Verification items for the finished model (mm, model axes). Coordinates: 2 decimals unless noted, no trailing zeros. Write each loop counter-clockwise with the first axis right and the second up, starting at its lowest first coordinate (ties: lowest second). Pieces come first, ordered by that corner, then holes. Notation, with made-up numbers: M -39,40 L -13,40 A6 ccw -13,45 Z; hole C 23,-18 d2. An arc over 180 degrees is marked long. One line per item, written item: value.
Autodesk Fusion 360 part; units mm, degrees
sketch "Sketch1" plane through (0, 0, 0) normal (0, 0, 1) x (1, 0, 0)
  line L0 (0, 0) -> (60, 0)
  line L1 (60, 0) -> (60, 60)
  line L2 (60, 60) -> (40, 60)
  line L3 (0, 0) -> (0, 20)
  line L4 (0, 20) -> (40, 60)
  dimension "d1" = 60
  dimension "d2" = 60
  dimension "d3" = 20
  dimension "d4" = 20
extrude "Extrude1" add sketch "Sketch1" along normal blind 4
hole "Hole2" at (10, 10, 4) direction (0, 0, -1) diameter 4.234 depth 34 tip angle 180
hole "Hole3" at (50, 10, 4) direction (0, 0, -1) diameter 4.234 depth 34 tip angle 180
hole "Hole4" at (50, 50, 4) direction (0, 0, -1) diameter 4.234 depth 34 tip angle 180
hole "Hole5" at (50, 30, 4) direction (0, 0, -1) diameter 4.234 depth 34 tip angle 180
hole "Hole6" at (30, 10, 4) direction (0, 0, -1) diameter 4.234 depth 34 tip angle 180
Item 1: Cross-section at D-D, the plane z = 2.05. Enter the section's corners in (x, y), and give its area (3 significant figures).
The answers:
outline: M 0,0 L 60,0 L 60,60 L 40,60 L 0,20 Z; hole C 10,10 d4.23; hole C 30,10 d4.23; hole C 50,10 d4.23; hole C 50,30 d4.23; hole C 50,50 d4.23
area: 2,730 mm²
Item 2: Draft check along Y on faces 1 (the face through (60, 30, 2)), 2 (the face through (51.878, 29.023, 1.972)), 3 (the face through (50, 60, 2)), 4 (the face through (9.907, 12.115, 1.972)). Enter one of: released by +Y, released by -Y, zero draft, split by the parting line, or undercut.
The answers:
face 1: zero draft
face 2: undercut
face 3: released by +Y
face 4: undercut
Item 3: Scan lines: line 1 (Y direction, x = 50, z = 1.2); line 2 (X direction, y = 9, z = 0.8). Record each from-to range of solid material in increasing order.
The answers:
line 1: y = 0 to 7.88, 12.12 to 27.88, 32.12 to 47.88, 52.12 to 60
line 2: x = 0 to 8.13, 11.87 to 28.13, 31.87 to 48.13, 51.87 to 60
Item 4: Cross-section at A-A, the plane x = 50. Enter the section's corners in (y, z).
The answers:
outline: M 0,0 L 7.88,0 L 7.88,4 L 0,4 Z; M 12.12,0 L 27.88,0 L 27.88,4 L 12.12,4 Z; M 32.12,0 L 47.88,0 L 47.88,4 L 32.12,4 Z; M 52.12,0 L 60,0 L 60,4 L 52.12,4 Z
Item 5: Cross-section at B-B, the plane y = 50. Enter the section's corners in (x, z).
The answers:
outline: M 30,0 L 47.88,0 L 47.88,4 L 30,4 Z; M 52.12,0 L 60,0 L 60,4 L 52.12,4 Z
